Geometry: final body of the model. Coordinates: model frame, mm. A direction names the side the tool comes from. Coordinates: 2 decimals unless noted, no trailing zeros. Order: outer loops, then holes, each group sorted by start corner. A loop starts at its lowest first (then second) coordinate and runs counter-clockwise, first axis right, second up. Notation, with made-up numbers: (51.25, 58) -> (106.25, 58) arc R18 ccw to (106.25, 75) -> close; hole circle Ø5 at (89.25, 71). An arc over 180 degrees is marked (long way). Use one line per item in the form item = value.
```python
from build123d import *

# Parameters (mm, degrees)
F0_W     = 88.9
F0_H     = 38.1
F1_DEPTH = 50.8
F2_W     = 63.5
F2_H     = 25.4
F3_DEPTH = 50.8
F4_W     = 25.4
F4_H     = 38.1
F5_DEPTH = 38.1
F6_R     = 6.35
F7_DEPTH = 25.4
F8_R     = 6.35
F9_DEPTH = 25.4


with BuildPart() as f1:
    # F0 (on Front) → F1 (new body)
    with BuildSketch(Plane.XZ):
        with Locations((1.052767, -5.984174)):
            Rectangle(F0_W, F0_H)
    extrude(amount=F1_DEPTH)

    # F2 (on face) → F3 (cut)
    with BuildSketch(Plane.XZ.offset(50.8)):
        with Locations((1.052767, 0.365826)):
            Rectangle(F2_W, F2_H)
    extrude(amount=-F3_DEPTH, mode=Mode.SUBTRACT)

    # F4 (on face) → F5 (cut)
    with BuildSketch(Plane.YZ.offset(45.502767)):
        with Locations((-38.1, -5.984174)):
            Rectangle(F4_W, F4_H)
    extrude(amount=-F5_DEPTH, mode=Mode.SUBTRACT)

    # F6 (on face) → F7 (cut)
    with BuildSketch(Plane.XY.offset(-12.334174)):
        with Locations((-17.997233, -38.1)):
            Circle(F6_R)
    extrude(amount=-F7_DEPTH, mode=Mode.SUBTRACT)

    # F8 (on face) → F9 (cut)
    with BuildSketch(Plane.XY.offset(-12.334174)):
        with Locations((7.402767, -12.7)):
            Circle(F8_R)
    extrude(amount=-F9_DEPTH, mode=Mode.SUBTRACT)


solid = f1.part
```
1) Contact query for flat-ended pins moving along their axis: P1, Ø19, axis at x = 30, z = -8.5, coming from the -Y side; P2, Ø8, axis at x = 15, y = -39, coming from the -Z side; P3, Ø6.5, axis at y = -33, z = -21.5, coming from the +X side; P4, Ø8, axis at x = 26, y = -27.5, coming from the -Z side. Output: stop coordinate, or through.
Results found:
P1 = -25.4
P2 = through
P3 = 7.4
P4 = -25.03
2) Pull-direction query (X, two-part tool) for faces 4 (the flat face through (-24, -50.8, -14)), 5 (the flat face through (45.503, -13, -6)), 6 (the flat face through (-30.697, -26, 0)), 7 (the cylindrical face through (-11.94, -36.19, -18.6)); classes: released by +X, released by -X, zero draft, split by the parting line, or undercut.
Results found:
face_4 = zero draft
face_5 = released by +X
face_6 = undercut
face_7 = undercut
3) Section A-A, the plane x = -18. Output: boundary loops of the cut face in (y, z), and give its area (3 significant figures).
Results found:
outline = (-50.8, -25.03) -> (-44.45, -25.03) -> (-44.45, -12.33) -> (-50.8, -12.33) -> close; (-31.75, -25.03) -> (0, -25.03) -> (0, -12.33) -> (-31.75, -12.33) -> close
area = 484 mm2
4) Section D-D, the plane z = -9.5. Output: boundary loops of the cut face in (x, y).
Results found:
outline = (-43.4, -50.8) -> (-30.7, -50.8) -> (-30.7, 0) -> (-43.4, 0) -> close; (32.8, -25.4) -> (45.5, -25.4) -> (45.5, 0) -> (32.8, 0) -> close
5) Section C-C, the plane z = -20.5. Output: boundary loops of the cut face in (x, y).
Results found:
outline = (-43.4, -50.8) -> (7.4, -50.8) -> (7.4, -25.4) -> (45.5, -25.4) -> (45.5, 0) -> (-43.4, 0) -> close; hole circle Ø12.7 at (-18, -38.1); hole circle Ø12.7 at (7.4, -12.7)
6) Section B-B, the plane y = -12.7. Output: boundary loops of the cut face in (x, z), and give its area (3 significant figures).
Results found:
outline = (-43.4, -25.03) -> (1.05, -25.03) -> (1.05, -12.33) -> (-30.7, -12.33) -> (-30.7, 13.07) -> (-43.4, 13.07) -> close; (13.75, -25.03) -> (45.5, -25.03) -> (45.5, 13.07) -> (32.8, 13.07) -> (32.8, -12.33) -> (13.75, -12.33) -> close
area = 1,610 mm2
7) Access query for faces 1 (the flat face through (7.403, -38, -19)), 2 (the flat face through (-6, -20, -12.334)), 3 (the flat face through (39, -13, 13.066)). Directions: +Z, -Z, +X, -X, +Y, -Y. A direction counts if a zero-diameter tool reaches every point of the face in a straight line with its end or side. Return the directions, or none.
Results found:
face_1 = +Z, -Z, +X, -Y
face_2 = +Z, +Y, -Y
face_3 = +Z, +X, -X, +Y, -Y
8) Material intervals for probe 1 along Z at (x, y) = (-3, -47.5); probe 2 along X at (y, z) = (-44.5, -12); probe 3 along Y at (x, z) = (3.5, -20), sorted ascending. Write a range as from..to.
Results found:
probe_1 = -25.03..-12.33
probe_2 = -43.4..-30.7
probe_3 = -50.8..-17.71, -7.69..0
